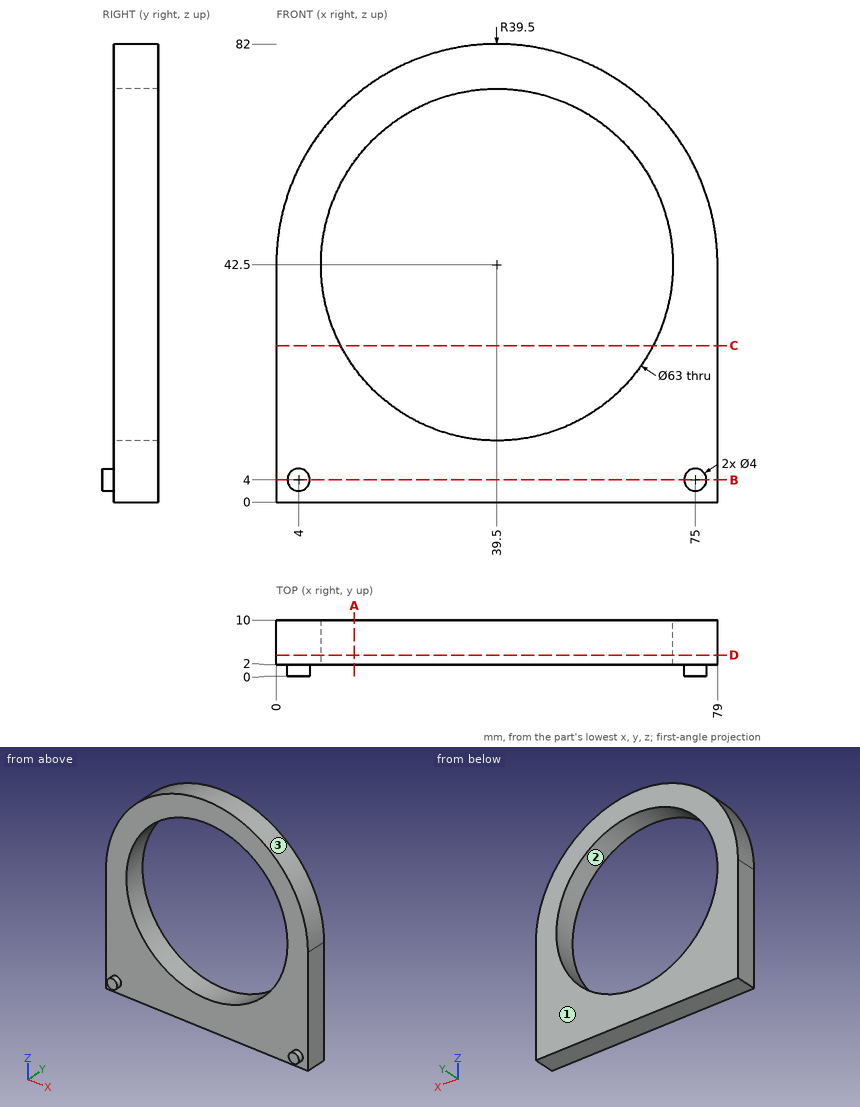
Drawing for the job (mm, zero at the part's lowest x, y, z). Round coordinates to 2 decimals unless told otherwise and drop trailing zeros. Write each loop counter-clockwise with the first axis right and the second up, starting at its lowest first coordinate (ties: lowest second). Pieces come first, ordered by that corner, then holes. Notation, with made-up numbers: M 68,-38.5 L 107,-38.5 A25 ccw 107,-7.5 Z; hole C 87.5,81 d5. An arc over 180 degrees is marked long. Answer in a Markdown table with one row per item.
1. Mould opens along X. For the marked faces 1, 2 and 3 say: +X half, -X half, draft (parallel to the pull), parting line (faces both ways), or undercut.
Geometry check:
| item | result |
|---|---|
| face 1 | draft |
| face 2 | undercut |
| face 3 | parting line |
2. Saw through at C-C (z = 28). List the corners of the cut face in (x, y), and give its area (3 significant figures).
Geometry check:
| item | result |
|---|---|
| outline | M 0,2 L 11.54,2 L 11.54,10 L 0,10 Z; M 67.46,2 L 79,2 L 79,10 L 67.46,10 Z |
| area | 185 mm2 |
3. Probe L1, parallel to Z at x = 39.5, y = 7.75; L2, parallel to X at y = 7.25, z = 42.5; L3, parallel to Y at x = 46.5, z = 3. List the from-to ranges inside material, lowest first. Write a range as [from, to].
Geometry check:
| item | result |
|---|---|
| L1 | [0, 11], [74, 82] |
| L2 | [0, 8], [71, 79] |
| L3 | [2, 10] |
4. Saw through at A-A (x = 14). List the corners of the cut face in (y, z), and give its area (3 significant figures).
Geometry check:
| item | result |
|---|---|
| outline | M 2,0 L 10,0 L 10,24.01 L 2,24.01 Z; M 2,60.99 L 10,60.99 L 10,72.67 L 2,72.67 Z |
| area | 285 mm2 |
5. Flat gauge pins, fed straight in: P1, Ø1, axis at x = 24, z = 11.5, coming from the -Y side; P2, Ø3, axis at y = 6, z = 70, coming from the +X side; P3, Ø1.5, axis at y = 6, z = 57, coming from the +X side. Where does each tip first touch, or does it go through?
Geometry check:
| item | result |
|---|---|
| P1 | y = 2 |
| P2 | x = 69.24 |
| P3 | x = 76.53 |
6. Saw through at D-D (y = 3.75). List the corners of the cut face in (x, z).
Geometry check:
| item | result |
|---|---|
| outline | M 0,0 L 79,0 L 79,42.5 A39.5 ccw 0,42.5 Z; hole C 39.5,42.5 d63 |
7. Saw through at B-B (z = 4). List the corners of the cut face in (x, y).
Geometry check:
| item | result |
|---|---|
| outline | M 0,2 L 2,2 L 2,0 L 6,0 L 6,2 L 73,2 L 73,0 L 77,0 L 77,2 L 79,2 L 79,10 L 0,10 Z |
